```python
from build123d import *

# Parameters (mm, degrees)
EXTRUDE_1_DEPTH     = 2.2
SKETCH_4_W          = 16
SKETCH_4_H          = 33.8
CUT_EXTRUDE_1_DEPTH = 1.2
F_2_0MM_1_D         = 4.5
FILLET_1_R          = 1.1
FILLET_2_R          = 8
FILLET_3_R          = 1


with BuildPart() as part:
    # 草圖2 → 填料-伸長1 (new body)
    with BuildSketch(Plane.XY):
        with BuildLine():
            Line((8, -18), (8, 15.8))
            Line((8, 15.8), (11.2, 15.8))
            Line((11.2, 15.8), (11.2, 36.703847577))
            Line((11.2, 36.703847577), (0.55, 42.852627944))
            ThreePointArc((0.55, 42.852627944), (0, 43), (-0.55, 42.852627944))
            Line((-0.55, 42.852627944), (-11.2, 36.703847577))
            Line((-11.2, 36.703847577), (-11.2, 15.8))
            Line((-11.2, 15.8), (-8, 15.8))
            Line((-8, 15.8), (-8, -18))
            Line((-8, -18), (8, -18))
        make_face()
        Polygon((8, 18), (-8, 18), (-9, 18), (-9, 35.433676985), (0, 40.629829408), (9, 35.433676985), (9, 18), align=None, mode=Mode.SUBTRACT)
    extrude(amount=EXTRUDE_1_DEPTH)

    # 草圖4 → 除料-伸長1 (cut)
    with BuildSketch(Plane.XY.offset(2.2)):
        with Locations((0, -1.1)):
            Rectangle(SKETCH_4_W, SKETCH_4_H)
    extrude(amount=-CUT_EXTRUDE_1_DEPTH, mode=Mode.SUBTRACT)

    # Ø2.0mm 定位孔1 (through all)
    with Locations(Plane(origin=(0, 7.5, 1), x_dir=(1, 0, 0), z_dir=(0, 0, 1))):
        with Locations((0, 0), (0, -17.2)):
            Hole(F_2_0MM_1_D / 2)

    # 圓角1
    fillet_1_edges = [part.edges().sort_by_distance(p)[0] for p in [
        (9, 35.433676985, 1.1),
        (0, 40.629829408, 1.1),
        (-9, 35.433676985, 1.1),
        (-9, 18, 1.1),
        (9, 18, 1.1),
        (-11.2, 15.8, 1.1),
        (-11.2, 36.703847577, 1.1),
        (11.2, 36.703847577, 1.1),
        (11.2, 15.8, 1.1),
    ]]
    fillet(fillet_1_edges, radius=FILLET_1_R)

    # 圓角2
    fillet_2_edges = [part.edges().sort_by_distance(p)[0] for p in [
        (8, -18, 0.5),
        (-8, -18, 0.5),
    ]]
    fillet(fillet_2_edges, radius=FILLET_2_R - 0.0001)  # a hair under: the kernel refuses the full size

    # 圓角3
    fillet_3_edges = [part.edges().sort_by_distance(p)[0] for p in [
        (-8, 15.8, 0.5),
        (8, 15.8, 0.5),
    ]]
    fillet(fillet_3_edges, radius=FILLET_3_R)


solid = part.part
```
Read the model definition and answer for the solid it produces. Units are mm, in the model's axes. A direction names the side the tool comes from. Give positions to 0.01 mm unless a question says otherwise; leave off trailing zeros. Order: outer loops, then holes, each group sorted by start corner. A loop starts at its lowest first (then second) coordinate and runs counter-clockwise, first axis right, second up. Notation, with made-up numbers: (85.25, -35.75) -> (130.25, -35.75) arc R18 cw to (130.25, -31.75) -> close; hole circle Ø6 at (14.5, -14). An arc over 180 degrees is marked (long way). One line per item, written item: value. Start each with the question number.
(1) The part is cut by section C-C (z = 0.45). State how many separate pieces and enclosed holes the cut face has, and give its area (3 significant figures).
(2) The part is cut by section A-A (y = 7.5). Determine the outline of the cut face in (x, z).
(3) Straight lines are drawn through the part: L1, parallel to Y at x = 0, z = 0.5; L2, parallel to X at y = 33, z = 1.25; L3, parallel to Y at x = -0.75, z = 0.7. For each, find the intervals that lie inside material, in ascending order.
(4) Flat-ended cylindrical pins translate along their axes: P1, Ø5.5, axis at x = -3.5, y = 5, coming from the +Z side; P2, Ø0.5, axis at y = 7, z = 0.5, coming from the +X side; P3, Ø1, axis at x = 2, z = 1.5, coming from the +Y side. Find the tip coordinate at first contact, or state that the pin passes through.
(5) A tool of negligible diameter and unlimited length cuts with its end or side. For faces 5 (the flat face through (0, -1, 1)), 6 (the flat face through (8, 2.2, 0.5)), 7 (the cylindrical face through (0, 43, 1)), 8 (the cylindrical face through (-5.594, -15.719, 0.507)), 9 (the cylindrical face through (-8.669, 18.314, 1.115)), from which of +Z, -Z, +X, -X, +Y, -Y can it reach the whole face along a straight path? Write none if from no direction.
(6) The part is cut by section B-B (x = -4). Determine the outline of the cut face in (y, z).
(7) The part is cut by section D-D (x = 1.25). Determine the outline of the cut face in (y, z).
(8) For a pull along X with two mould halves and no side action, classify faces 1 (the cylindrical face through (-1.21, 9.397, 0.493)), 2 (the cylindrical face through (0.29, -7.47, 0.49)), 3 (the flat face through (2, 6, 0)), 4 (the cylindrical face through (-8.301, 15.515, 0.507)) as released by +X, released by -X, zero draft, split by the parting line, or undercut.
Taken from the geometry:
1. separate pieces: 1
1. enclosed holes: 3
1. area: 662 mm^2
2. outline: (-8, 0) -> (-2.25, 0) -> (-2.25, 1) -> (-8, 1) -> close; (2.25, 0) -> (8, 0) -> (8, 1) -> (2.25, 1) -> close
3. L1: -18 to -11.95, -7.45 to 5.25, 9.75 to 18, 40.46 to 43
3. L2: -11.2 to -9, 9 to 11.2
3. L3: -17.96 to -11.82, -7.58 to 5.38, 9.62 to 18, 40.2 to 42.74
4. P1: z = 1
4. P2: x = 8
4. P3: y = 42.3
5. face 5: +Z, +X, -X, -Y
5. face 6: +Z, -Z, +X, -Y
5. face 7: +Z, -Z, +Y
5. face 8: +Z, -Z, -X, -Y
5. face 9: +Z, -Z
6. outline: (-16.93, 0) -> (18, 0) -> (18, 2.2) -> (15.8, 2.2) -> (15.8, 1) -> (-16.93, 1) -> close; (38.32, 0) -> (40.86, 0) -> (40.86, 2.2) -> (38.32, 2.2) -> close
7. outline: (-17.9, 0) -> (-11.57, 0) -> (-11.57, 1) -> (-17.9, 1) -> close; (-7.83, 0) -> (5.63, 0) -> (5.63, 1) -> (-7.83, 1) -> close; (9.37, 0) -> (18, 0) -> (18, 2.2) -> (15.8, 2.2) -> (15.8, 1) -> (9.37, 1) -> close; (39.91, 0) -> (42.45, 0) -> (42.45, 2.2) -> (39.91, 2.2) -> close
8. face 1: undercut
8. face 2: undercut
8. face 3: zero draft
8. face 4: released by -X
